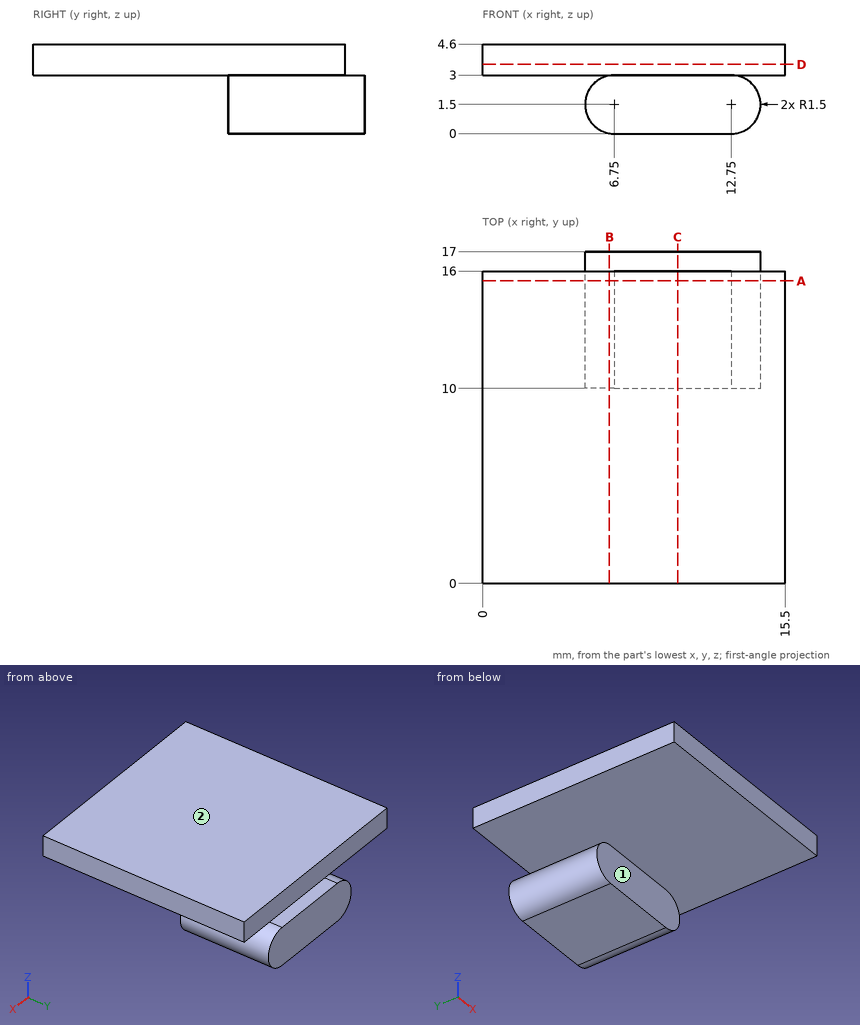
Can you work these out from the drawing? Everything is in mm from the part's minimum corner. A direction names the side the tool comes from. Round coordinates to 2 decimals unless told otherwise and drop trailing zeros. Write each loop counter-clockwise with the first axis right and the second up, starting at its lowest first coordinate (ties: lowest second). Pieces come first, ordered by that corner, then holes. Notation, with made-up numbers: (0, 59.25) - (29, 59.25) arc R17 ccw to (29, 83.25) - close; hole circle Ø7 at (-18.75, 42.5). An arc over 180 degrees is marked (long way). Put each result on its own line as item: value. Start each with the question number.
(1) I need wall thicknesses on probe 1 along Z at (x, y) = (1, 6.5); probe 2 along Y at (x, z) = (5.25, 4.4); probe 3 along Y at (x, z) = (10.25, 2.15). Which ranges of each line are inside material? Lowest first, please.
(2) I want a section at D-D, the plane z = 3.55. Please give me the cut outline in (x, y).
(3) Will these pins go through, and if not, where does the flat tip stop? pin 1 (0.8 mm diameter, centred on x = 11.5, z = 3.5, fed in from +Y); pin 2 (1.5 mm diameter, centred on x = 11.5, z = 2, fed in from -Y); pin 3 (8 mm diameter, centred on x = 9, y = 5, fed in from -Z).
(4) I want a section at C-C, the plane x = 10. Please give me the cut outline in (y, z), plus the area to 3 significant figures.
(5) For the marked faces 1 and 2, which set-ups out of +Z, -Z, +X, -X, +Y, -Y let a thin tool reach every point of the face, with its end or its side?
(6) I want a section at B-B, the plane x = 6.5. Please give me the cut outline in (y, z), plus the area to 3 significant figures.
(7) I want a section at A-A, the plane y = 15.5. Please give me the cut outline in (x, z), plus the area to 3 significant figures.
Here are the results:
1. probe 1: z = 3 to 4.6
1. probe 2: y = 0 to 16
1. probe 3: y = 10 to 17
2. outline: (0, 0) - (15.5, 0) - (15.5, 16) - (0, 16) - close
3. pin 1: stops at y = 16
3. pin 2: stops at y = 10
3. pin 3: stops at z = 3
4. outline: (0, 3) - (10, 3) - (10, 0) - (17, 0) - (17, 3) - (16, 3) - (16, 4.6) - (0, 4.6) - close
4. area: 46.6 mm^2
5. face 1: -Z, +X, -X, -Y
5. face 2: +Z, +X, -X, +Y, -Y
6. outline: (0, 3) - (16, 3) - (16, 4.6) - (0, 4.6) - close; (10, 0.02) - (17, 0.02) - (17, 2.98) - (10, 2.98) - close
6. area: 46.3 mm^2
7. outline: (0, 3) - (6.75, 3) arc R1.5 ccw to (6.75, 0) - (12.75, 0) arc R1.5 ccw to (12.75, 3) - (15.5, 3) - (15.5, 4.6) - (0, 4.6) - close
7. area: 49.9 mm^2
